The figure shows three views and two pictorial views of one solid part (mm, origin at its lowest corner). Answer the questions. Coordinates: 2 decimals unless noted, no trailing zeros. Loops run counter-clockwise (first coordinate to the right, second up) from the corner with the lowest first, then second, coordinate; pieces in that order, holes last. Notation, with made-up numbers: (38, -9) -> (94, -9) arc R24 cw to (94, 15) -> close; hole circle Ø9 at (-23, 59). An arc over 180 degrees is marked (long way). Answer in a Markdown table with one row per item.
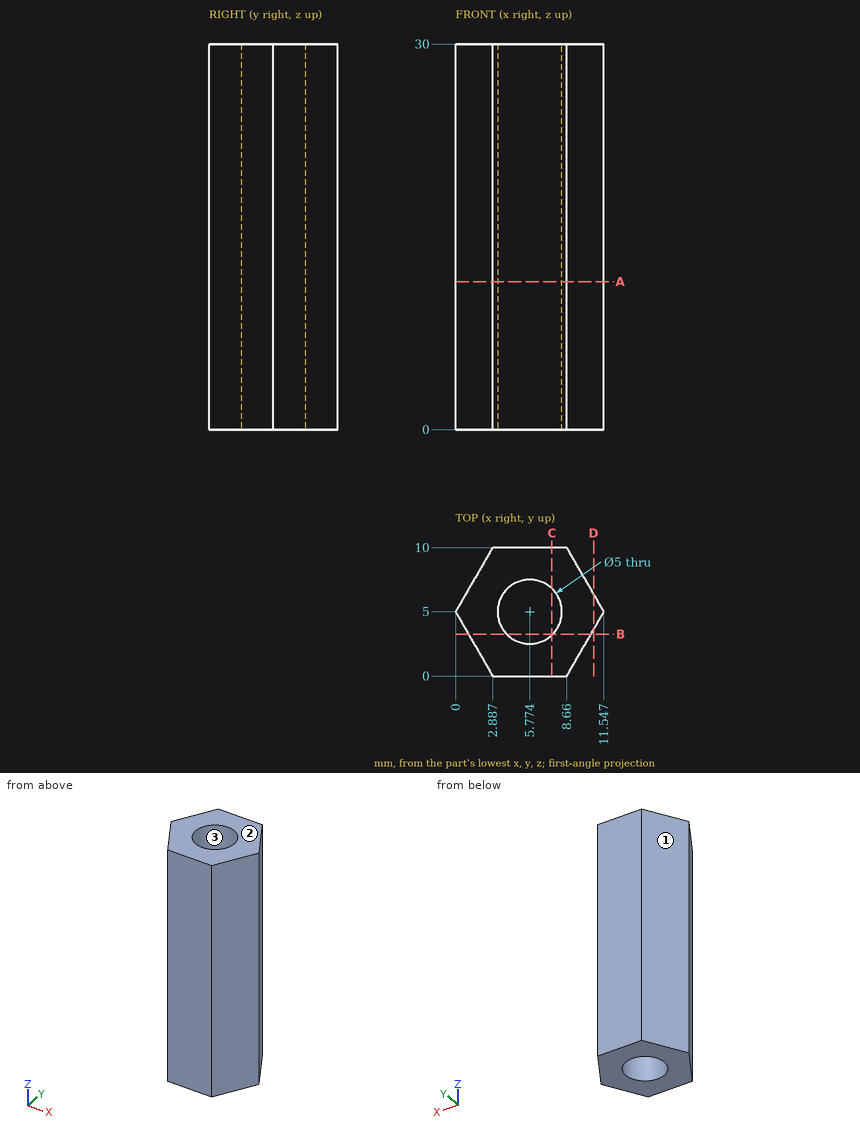
Item 1: A cutting plane is placed at B-B, the plane y = 3.25. Determine the outline of the cut face in (x, z), plus the area to 3 significant figures.
Findings below:
| item | result |
|---|---|
| outline | (1.01, 0) -> (3.99, 0) -> (3.99, 30) -> (1.01, 30) -> close; (7.56, 0) -> (10.54, 0) -> (10.54, 30) -> (7.56, 30) -> close |
| area | 179 mm2 |
Item 2: Flat-ended cylindrical pins translate along their axes: pin 1 Ø1 at (x, y) = (10.5, 1.5) entering from +Z; pin 2 Ø2 at (x, z) = (2, 25) entering from +Y; pin 3 Ø3 at (y, z) = (2, 18.5) entering from -X (1 decimal). Find the tip coordinate at first contact, or state that the pin passes through.
Findings below:
| item | result |
|---|---|
| pin 1 | passes through |
| pin 2 | stops at y = 10 |
| pin 3 | stops at x = 0.9 |
Item 3: Determine the mould class of the marked faces 1, 2 and 3 for opening direction Y: +Y half, -Y half, draft (parallel to the pull), parting line (faces both ways), or undercut.
Findings below:
| item | result |
|---|---|
| face 1 | +Y half |
| face 2 | draft |
| face 3 | undercut |
Item 4: Find the intervals of material crossed by probe 1 along X at (y, z) = (4, 10.25) (1 decimal); probe 2 along X at (y, z) = (5.5, 24.25) (1 decimal); probe 3 along Y at (x, z) = (4.5, 20.75), in increasing order.
Findings below:
| item | result |
|---|---|
| probe 1 | x = 0.6 to 3.5, 8.1 to 11 |
| probe 2 | x = 0.3 to 3.3, 8.2 to 11.3 |
| probe 3 | y = 0 to 2.85, 7.15 to 10 |
Item 5: A cutting plane is placed at C-C, the plane x = 7.5. Determine the outline of the cut face in (y, z).
Findings below:
| item | result |
|---|---|
| outline | (0, 0) -> (3.19, 0) -> (3.19, 30) -> (0, 30) -> close; (6.81, 0) -> (10, 0) -> (10, 30) -> (6.81, 30) -> close |
Item 6: A cutting plane is placed at A-A, the plane z = 11.5. Determine the outline of the cut face in (x, y).
Findings below:
| item | result |
|---|---|
| outline | (0, 5) -> (2.89, 0) -> (8.66, 0) -> (11.55, 5) -> (8.66, 10) -> (2.89, 10) -> close; hole circle Ø5 at (5.77, 5) |
Item 7: A cutting plane is placed at D-D, the plane x = 10.75. Determine the outline of the cut face in (y, z).
Findings below:
| item | result |
|---|---|
| outline | (3.62, 0) -> (6.38, 0) -> (6.38, 30) -> (3.62, 30) -> close |
